Input: part model. Units: mm. Frame: model coordinates. A direction names the side the tool comes from. Coordinates: 2 decimals unless noted, no trailing zeros. Order: outer loops, then holes, each group sorted by start corner. A loop starts at its lowest first (then second) coordinate and runs counter-clockwise, first axis right, second up. Notation, with made-up numbers: M 42.5,-12.75 L 80.5,-12.75 A33 cw 80.5,23.25 Z; hole C -7.75,-2.5 d2. An arc over 180 degrees is marked long. Answer in a Markdown table with one row per item.
Autodesk Inventor part; units mm, degrees
ref_plane "YZ Plane" through (0, 0, 0) normal (1, 0, 0) x (0, 1, 0)
ref_plane "XZ Plane" through (0, 0, 0) normal (0, 1, 0) x (-1, 0, 0)
ref_plane "XY Plane" through (0, 0, 0) normal (0, 0, 1) x (1, 0, 0)
sketch "スケッチ3" plane through (0, 0, 0) normal (0, 0, 1) x (1, 0, 0)
  line L0 (43.5, -28.5) -> (-43.5, -28.5)
  line L1 (-43.5, -28.5) -> (-43.5, 28.5)
  line L2 (-43.5, 28.5) -> (43.5, 28.5)
  line L3 (43.5, 28.5) -> (43.5, -28.5)
  line L4 (43.5, -28.5) -> (-43.5, 28.5) construction
  line L5 (-43.5, -28.5) -> (43.5, 28.5) construction
  point P0 (0, 0)
  dimension "d4" = 57
  dimension "d5" = 87
extrude "枠" add sketch "スケッチ3" along normal blind 70
sketch "スケッチ4" plane through (0, 0, 0) normal (0, 0, -1) x (-1, 0, 0)
  line L0 (40.6, -26.5) -> (-40.6, -26.5)
  line L1 (-40.6, -26.5) -> (-40.6, 26.5)
  line L2 (-40.6, 26.5) -> (40.6, 26.5)
  line L3 (40.6, 26.5) -> (40.6, -26.5)
  line L4 (40.6, -26.5) -> (-40.6, 26.5) construction
  line L5 (-40.6, -26.5) -> (40.6, 26.5) construction
  point P0 (0, 0)
  dimension "d8" = 81.2
  dimension "d9" = 53
extrude "本体" cut sketch "スケッチ4" against normal blind 56
sketch "スケッチ5" plane through (-43.5, 28.5, 0) normal (0, 1, 0) x (1, 0, 0)
  line L0 (0, 0) -> (0, -70)
  line L1 (87, 0) -> (87, -70)
  line L2 (0, -51) -> (87, -51)
  line L3 (87, -51) -> (87, -55)
  line L4 (87, -55) -> (0, -55)
  line L5 (0, -55) -> (0, -51)
  line L6 (87, -70) -> (0, -70)
  point P0 (43.5, 0)
  dimension "d12" = 15
  dimension "d13" = 4
extrude "台" add sketch "スケッチ5" against normal blind 55 contours L2 L1 L4 L0
sketch "スケッチ6" plane through (0, 0, 0) normal (0, 0, -1) x (-1, 0, 0)
  line L0 (40.6, -26.5) -> (40.6, 26.5)
  line L1 (43.1, 19.5) -> (40.6, 19.5)
  line L2 (40.6, 19.5) -> (40.6, 13.5)
  line L3 (40.6, 13.5) -> (43.1, 13.5)
  line L4 (43.1, 13.5) -> (43.1, 19.5)
  line L5 (40.6, 26.5) -> (-40.6, 26.5)
  line L6 (32.6, 26.5) -> (26.6, 26.5)
  line L7 (26.6, 26.5) -> (26.6, 28)
  line L8 (26.6, 28) -> (32.6, 28)
  line L9 (32.6, 28) -> (32.6, 26.5)
  line L10 (-26.6, 26.5) -> (-32.6, 26.5)
  line L11 (-32.6, 26.5) -> (-32.6, 28)
  line L12 (-32.6, 28) -> (-26.6, 28)
  line L13 (-26.6, 28) -> (-26.6, 26.5)
  line L14 (-40.6, -26.5) -> (-40.6, 26.5)
  point P0 (0, 0)
  dimension "d16" = 2.5
  dimension "d17" = 13
  dimension "d18" = 6
  dimension "d19" = 1.5
  dimension "d20" = 8
  dimension "d21" = 6
  dimension "d22" = 1.5
  dimension "d23" = 6
  dimension "d24" = 8
extrude "溝" cut sketch "スケッチ6" against normal blind 51
sketch "スケッチ7" plane through (40.6, -26.5, 0) normal (-1, 0, 0) x (0, 0, 1)
  line L0 (51, 10) -> (31, 10)
  line L1 (31, 10) -> (31, 43)
  line L2 (31, 43) -> (51, 43)
  line L3 (51, 43) -> (51, 10)
  line L4 (51, 53) -> (0, 53)
  line L5 (51, 0) -> (51, 53)
  point P0 (0, 26.5)
  point P1 (0, 0)
  dimension "d27" = 10
  dimension "d28" = 10
  dimension "d29" = 20
  dimension "d30" = 0
extrude "USB穴" cut sketch "スケッチ7" along normal through all both and the other way through all
sketch "スケッチ8" plane through (-26.6, 26.5, 0) normal (0, -1, 0) x (1, 0, 0)
  line L0 (67.2, 51) -> (-14, 51)
  line L1 (48.2, 31) -> (5, 31)
  line L2 (5, 31) -> (5, 51)
  line L3 (5, 51) -> (48.2, 51)
  line L4 (48.2, 51) -> (48.2, 31)
  line L5 (53.2, 0) -> (53.2, 51)
  line L6 (0, 51) -> (0, 0)
  point P0 (26.6, 0)
  dimension "d33" = 5
  dimension "d34" = 5
  dimension "d35" = 20
extrude "ボタン押下用穴" cut sketch "スケッチ8" along normal through all both and the other way through all
sketch "su" plane through (-32.6, 26.5, 51) normal (0, 0, -1) x (-1, 0, 0)
  line L0 (-64.2, -53) -> (-61.7, -53)
  line L1 (-61.7, -53) -> (-61.7, -52)
  line L2 (-61.7, -52) -> (-64.2, -52)
  line L3 (-64.2, -52) -> (-64.2, -53)
  line L4 (-3.5, -53) -> (-1, -53)
  line L5 (-1, -53) -> (-1, -52)
  line L6 (-1, -52) -> (-3.5, -52)
  line L7 (-3.5, -52) -> (-3.5, -53)
  line L8 (-74.2, -22.5) -> (-73.2, -22.5)
  line L9 (-73.2, -22.5) -> (-73.2, -20)
  line L10 (-73.2, -20) -> (-74.2, -20)
  line L11 (-74.2, -20) -> (-74.2, -22.5)
  line L12 (-73.2, -53) -> (-73.2, -43)
  line L13 (8, -53) -> (-73.2, -53)
  line L14 (8, -13) -> (8, -53)
  point P0 (-32.6, -26.5)
  point P1 (-65.2, 0)
  point P2 (8, -40)
  dimension "d49" = 9
  dimension "d50" = 0
  dimension "d51" = 2.5
  dimension "d52" = 1
  dimension "d53" = 20
  dimension "d54" = 1
  dimension "d56" = 2.5
  dimension "d57" = 9
  dimension "d58" = 1
  dimension "d59" = 2.5
  dimension "d60" = 0
extrude "凸" add sketch "su" along normal blind 3
sketch "スケッチ11" plane through (0, 0, 70) normal (0, 0, 1) x (1, 0, 0)
  line L0 (43.5, -28.5) -> (-43.5, -28.5)
  line L1 (43.5, 28.5) -> (-43.5, 28.5)
  line L2 (-43.5, -28.5) -> (43.5, -28.5)
  line L3 (43.5, -28.5) -> (43.5, 28.5)
  line L4 (43.5, 28.5) -> (-43.5, 28.5)
  line L5 (-43.5, 28.5) -> (-43.5, -28.5)
  point P0 (0, 0)
extrude "底面" add sketch "スケッチ11" against normal up to surface (15 mm away)
sketch "スケッチ13" plane through (-43.5, -28.5, 0) normal (0, -1, 0) x (1, 0, 0)
  line L0 (87, 0) -> (87, 70)
  line L1 (87, 53) -> (72, 53)
  line L2 (72, 53) -> (72, 68)
  line L3 (72, 68) -> (87, 68)
  line L4 (87, 68) -> (87, 53)
  line L5 (0, 0) -> (0, 70)
  line L6 (0, 53) -> (15, 53)
  line L7 (15, 53) -> (15, 68)
  line L8 (15, 68) -> (0, 68)
  line L9 (0, 68) -> (0, 53)
  line L10 (0, 70) -> (87, 70)
  point P0 (43.5, 0)
  dimension "d70" = 2
  dimension "d71" = 15
  dimension "d72" = 15
  dimension "d73" = 15
extrude "ネジ止め1" cut sketch "スケッチ13" against normal blind 15
sketch "スケッチ14" plane through (-43.5, 28.5, 0) normal (0, 1, 0) x (1, 0, 0)
  line L0 (0, 0) -> (0, -70)
  line L1 (0, -53) -> (15, -53)
  line L2 (15, -53) -> (15, -68)
  line L3 (15, -68) -> (0, -68)
  line L4 (0, -68) -> (0, -53)
  line L5 (87, 0) -> (87, -53)
  line L6 (87, -53) -> (72, -53)
  line L7 (72, -53) -> (72, -68)
  line L8 (72, -68) -> (87, -68)
  line L9 (87, -68) -> (87, -53)
  line L10 (87, -70) -> (0, -70)
  point P0 (43.5, 0)
  dimension "d76" = 15
  dimension "d77" = 15
  dimension "d78" = 15
  dimension "d79" = 2
extrude "ネジ止め2" cut sketch "スケッチ14" against normal blind 15
sketch "スケッチ19" plane through (0, 0, 0) normal (0, 0, -1) x (-1, 0, 0)
  line L0 (-43.5, 28.5) -> (43.5, 28.5)
  line L1 (-43.5, -28.5) -> (-28.5, -28.5)
  line L2 (43.5, 28.5) -> (-43.5, 28.5)
  line L3 (-43.5, 28.5) -> (-43.5, -28.5)
  line L4 (-43.5, -28.5) -> (43.5, -28.5)
  line L5 (43.5, -28.5) -> (43.5, 28.5)
  point P0 (0, 0)
extrude "上面削り" cut sketch "スケッチ19" against normal blind 42
sketch "ネジ穴用" plane through (0, 0, 70) normal (0, 0, 1) x (1, 0, 0)
  line L0 (37.5, 17.5) -> (-38.5, 17.5)
  line L1 (-38.5, 17.5) -> (-38.5, -21.5)
  line L2 (-38.5, -21.5) -> (37.5, -21.5)
  line L3 (37.5, -21.5) -> (37.5, 17.5)
  line L4 (43.5, -28.5) -> (43.5, 28.5)
  line L5 (-43.5, -28.5) -> (43.5, -28.5)
  point P0 (0, 0)
  dimension "d100" = 39
  dimension "d101" = 76
  dimension "d102" = 6
  dimension "d103" = 7
sketch "スケッチ23" plane through (0, 0, 42) normal (0, 0, -1) x (-1, 0, 0)
  line L0 (-32.6, 26.5) -> (-32.6, 28)
  line L1 (-26.6, 28) -> (-26.6, 26.5)
  line L2 (-32.6, 28.5) -> (-26.6, 28.5)
  line L3 (-26.6, 28.5) -> (-26.6, 26.5)
  line L4 (-26.6, 26.5) -> (-32.6, 26.5)
  line L5 (-32.6, 26.5) -> (-32.6, 28.5)
  line L6 (26.6, 28) -> (26.6, 26.5)
  line L7 (32.6, 26.5) -> (32.6, 28)
  line L8 (26.6, 26.5) -> (32.6, 26.5)
  line L9 (32.6, 26.5) -> (32.6, 28.5)
  line L10 (32.6, 28.5) -> (26.6, 28.5)
  line L11 (26.6, 28.5) -> (26.6, 26.5)
  point P0 (0, 0)
  point P1 (26.6, 28.5)
extrude "押し出し18" add sketch "スケッチ23" against normal blind 2
hole "穴2" at (-38.5, -21.5, 70) at (37.5, -21.5, 70) at (37.5, 17.5, 70) at (-38.5, 17.5, 70) direction (0, 0, -1) diameter 3 depth 4 tip angle 118
properties part number "cmoda7"
1) Material intervals for probe 1 along X at (y, z) = (-21.5, 69); probe 2 along Y at (x, z) = (37.5, 68.45); probe 3 along Y at (x, z) = (-40, 45.5), sorted ascending.
Resolved:
| item | result |
|---|---|
| probe 1 | x = -43.5 to -40, -37 to 36, 39 to 43.5 |
| probe 2 | y = -28.5 to -23, -20 to 16, 19 to 28.5 |
| probe 3 | y = -28.5 to -26.5, 26.5 to 28.5 |
2) Reachability of faces 1 (the face through (-43.1, 18, 46)), 2 (the face through (-37.6, -20.3, 69)), 3 (the face through (-36, 21, 53)), 4 (the face through (36, 13.5, 60)), 5 (the face through (21.6, 28, 47)) from +Z, -Z, +X, -X, +Y, -Y: full face, straight path, thin tool, end or side. Return the list, or none.
Resolved:
| item | result |
|---|---|
| face 1 | -Z |
| face 2 | +Z |
| face 3 | -X, +Y |
| face 4 | +X, +Y |
| face 5 | -Z, +Y, -Y |
3) Mould query, pull axis Y, two halves, no side actions, for faces 6 (the face through (36, -13.5, 61)), 7 (the face through (43.5, 0, 56)), 8 (the face through (-33, 26.5, 46)), 9 (the face through (-30, -25.5, 50)). Classes: +Y half, -Y half, draft (parallel to the pull), parting line (faces both ways), or undercut.
Resolved:
| item | result |
|---|---|
| face 6 | -Y half |
| face 7 | draft |
| face 8 | undercut |
| face 9 | undercut |
4) Cut plane A-A, the plane z = 47. State how many separate pieces and enclosed holes the cut face has, and give its area (3 significant figures).
Resolved:
| item | result |
|---|---|
| separate pieces | 4 |
| enclosed holes | 0 |
| area | 266 mm2 |
5) Contact query for flat-ended pins moving along their axis: pin 1 (8 mm diameter, centred on x = 33.5, z = 66.5, fed in from +Y); pin 2 (4.5 mm diameter, centred on x = 33, z = 63, fed in from +Y); pin 3 (12 mm diameter, centred on x = -7.5, y = -4, fed in from -Z); pin 4 (4.5 mm diameter, centred on x = 35.5, z = 64, fed in from -Y). Output: stop coordinate, or through.
Resolved:
| item | result |
|---|---|
| pin 1 | stops at y = 28.5 |
| pin 2 | stops at y = 13.5 |
| pin 3 | stops at z = 51 |
| pin 4 | stops at y = -13.5 |
6) Cut plane B-B, the plane x = -38.5. Output: boundary loops of the cut face in (y, z), and give its area (3 significant figures).
Resolved:
| item | result |
|---|---|
| outline | M -28.5,42 L -26.5,42 L -26.5,51 L 26.5,51 L 26.5,42 L 28.5,42 L 28.5,53 L 13.5,53 L 13.5,68 L 16,68 L 16,70 L -20,70 L -20,68 L -13.5,68 L -13.5,53 L -28.5,53 Z; M -28.5,68 L -23,68 L -23,70 L -28.5,70 Z; M 19,68 L 28.5,68 L 28.5,70 L 19,70 Z |
| area | 657 mm2 |
7) Cut plane D-D, the plane z = 54.25. Output: boundary loops of the cut face in (x, y).
Resolved:
| item | result |
|---|---|
| outline | M -43.5,-13.5 L -28.5,-13.5 L -28.5,-28.5 L 28.5,-28.5 L 28.5,-13.5 L 43.5,-13.5 L 43.5,13.5 L 28.5,13.5 L 28.5,28.5 L -28.5,28.5 L -28.5,13.5 L -43.5,13.5 Z |
8) Cut plane C-C, the plane y = 17.5. Output: boundary loops of the cut face in (x, z), and give its area (3 significant figures).
Resolved:
| item | result |
|---|---|
| outline | M -43.5,42 L -43.1,42 L -43.1,51 L 40.6,51 L 40.6,42 L 43.5,42 L 43.5,53 L 28.5,53 L 28.5,68 L 36,68 L 36,70 L -37,70 L -37,68 L -28.5,68 L -28.5,53 L -43.5,53 Z; M -43.5,68 L -40,68 L -40,70 L -43.5,70 Z; M 39,68 L 43.5,68 L 43.5,70 L 39,70 Z |
| area | 1,220 mm2 |
